The listing builds one solid part. Answer for the finished solid, in the listing's coordinates (mm). Give positions to 0.01 mm unless a question says otherwise; leave off trailing zeros. Order: outer loops, then holes, each group sorted by start corner. A loop starts at its lowest first (then second) coordinate and runs counter-clockwise, first axis right, second up. Notation, with made-up numbers: (-7.5, -23) - (25.5, -23) arc R9 ccw to (25.5, -18) - close; hole circle Ø4 at (71.5, 72.5). An arc over 180 degrees is marked (long way). Answer in a Markdown table with one row per item.
from build123d import *

# Parameters (mm, degrees)
SKETCH1_R              = 247.65
SKETCH1_R_2            = 73.025
BOSS_EXTRUDE1_DEPTH    = 6.35
SKETCH3_R              = 11
CUT_EXTRUDE1_DEPTH     = 7.35
F_10_32_TAPPED_HOLE1_D = 4.0386
SKETCH8_R              = 3.2512
CUT_EXTRUDE2_DEPTH     = 7.35
SKETCH9_R              = 3.2639
CUT_EXTRUDE3_DEPTH     = 7.35
CIRPATTERN1_COUNT      = 5


with BuildPart() as part:
    # Sketch1 → Boss-Extrude1 (new body)
    with BuildSketch(Plane(origin=(0, 0, 0), x_dir=(1, 0, 0), z_dir=(0, 1, 0))):
        Circle(SKETCH1_R)
        with Locations((0, 158.75)):
            Circle(SKETCH1_R_2, mode=Mode.SUBTRACT)
        with Locations((150.980221962, 49.056447857)):
            Circle(SKETCH1_R_2, mode=Mode.SUBTRACT)
        with Locations((93.310908801, -128.431447857)):
            Circle(SKETCH1_R_2, mode=Mode.SUBTRACT)
        with Locations((-93.310908801, -128.431447857)):
            Circle(SKETCH1_R_2, mode=Mode.SUBTRACT)
        with Locations((-150.980221962, 49.056447857)):
            Circle(SKETCH1_R_2, mode=Mode.SUBTRACT)
    extrude(amount=BOSS_EXTRUDE1_DEPTH)

    # Sketch3 → Cut-Extrude1 (cut, through all)
    with BuildSketch(Plane(origin=(-5.184519995, 6.35, -2.448578058), x_dir=(1, 0, 0), z_dir=(0, 1, 0))):
        with Locations((5.184519995, -2.448578058)):
            Circle(SKETCH3_R)
    extrude(amount=-CUT_EXTRUDE1_DEPTH, mode=Mode.SUBTRACT)

    # #10-32 Tapped Hole1 (through all)
    with Locations(Plane(origin=(-5.184519995, 6.35, -2.448578058), x_dir=(1, 0, 0), z_dir=(0, 1, 0))):
        with Locations((-3.546730005, 12.674390556), (13.915769995, 12.674390556), (22.647019995, -2.448578058), (13.915769995, -17.571546671), (-3.546730005, -17.571546671), (-12.277980005, -2.448578058)):
            Hole(F_10_32_TAPPED_HOLE1_D / 2)

    # Sketch8 → Cut-Extrude2 (cut, through all)
    with BuildSketch(Plane(origin=(0, 6.35, 0), x_dir=(1, 0, 0), z_dir=(0, 1, 0))):
        with Locations((0, -234.95)):
            Circle(SKETCH8_R)
        with Locations((-223.450728504, -72.603542828)):
            Circle(SKETCH8_R)
        with Locations((-138.100145026, 190.078542828)):
            Circle(SKETCH8_R)
        with Locations((138.100145026, 190.078542828)):
            Circle(SKETCH8_R)
        with Locations((223.450728504, -72.603542828)):
            Circle(SKETCH8_R)
    extrude(amount=-CUT_EXTRUDE2_DEPTH, mode=Mode.SUBTRACT)

    # Sketch9 → Cut-Extrude3 (cut, through all)
    with BuildSketch(Plane(origin=(0, 6.35, 0), x_dir=(1, 0, 0), z_dir=(0, 1, 0))):
        with Locations((0, -95.3389)):
            Circle(SKETCH9_R)
    cut_extrude3 = extrude(amount=-CUT_EXTRUDE3_DEPTH, mode=Mode.SUBTRACT)

    # CirPattern1: Cut-Extrude3 ×5 about axis
    cirpattern1_axis = Axis((0, 0, 0), (0, 1, 0))
    for i in range(1, CIRPATTERN1_COUNT):
        add(cut_extrude3.rotate(cirpattern1_axis, i * 360 / CIRPATTERN1_COUNT), mode=Mode.SUBTRACT)


solid = part.part
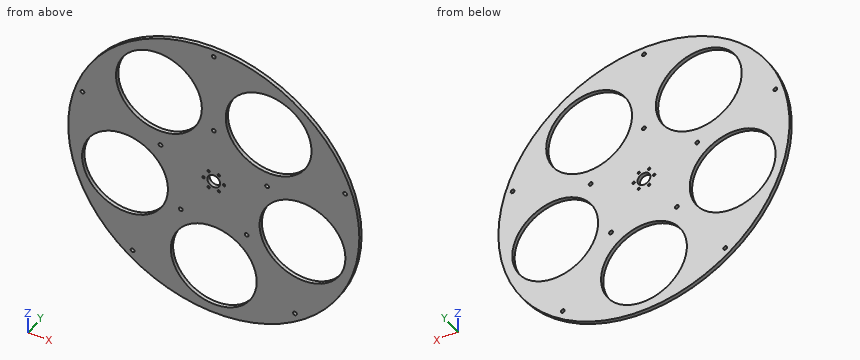
Item 1: Find section B-B on x = 120.5. Write down the section's boundary in (y, z).
Answer block:
| item | result |
|---|---|
| outline | (0, -216.36) - (6.35, -216.36) - (6.35, -115.42) - (0, -115.42) - close; (0, 17.3) - (6.35, 17.3) - (6.35, 60.66) - (0, 60.66) - close; (0, 196.21) - (6.35, 196.21) - (6.35, 216.36) - (0, 216.36) - close |
Item 2: Find section A-A on z = -206.5. Write down the section's boundary in (x, y).
Answer block:
| item | result |
|---|---|
| outline | (-136.71, 0) - (-55.25, 0) - (-55.25, 6.35) - (-136.71, 6.35) - close; (55.25, 0) - (136.71, 0) - (136.71, 6.35) - (55.25, 6.35) - close |
Item 3: Find section C-C on x = -181.5. Write down the section's boundary in (y, z), then the cut area to 3 significant figures.
Answer block:
| item | result |
|---|---|
| outline | (0, -168.49) - (6.35, -168.49) - (6.35, -115.4) - (0, -115.4) - close; (0, 17.29) - (6.35, 17.29) - (6.35, 168.49) - (0, 168.49) - close |
| area | 1,300 mm² |
Item 4: Consider line 1 (Z direction, x = 0, y = 2.75) (3 decimals); line 2 (X direction, y = 5, z = 7); line 3 (X direction, y = 4.75, z = 178). Determine where each line is inside the solid, lowest interval first.
Answer block:
| item | result |
|---|---|
| line 1 | -247.65 to -231.775, -85.725 to -11, 11 to 92.075, 98.603 to 231.699, 238.201 to 247.65 |
| line 2 | -247.55 to -197.78, -104.18 to -8.49, 8.49 to 104.18, 197.78 to 247.55 |
| line 3 | -172.18 to -146.94, -39.69 to 39.69, 146.94 to 172.18 |
Item 5: Find section D-D on y = 3.5. Count the separate pieces of the cut face and the enclosed holes in it, then the cut area to 3 significant figures.
Answer block:
| item | result |
|---|---|
| separate pieces | 1 |
| enclosed holes | 22 |
| area | 108,000 mm² |
Item 6: This flat-tipped pin is pushed along its axis until it touches: P1, Ø3, axis at y = 1, z = 54.5, coming from the +X side. Where does it stop, or does it pass through?
Answer block:
| item | result |
|---|---|
| P1 | x = 241.91 |
